Read the model definition and answer for the solid it produces. Units are mm, in the model's axes. A direction names the side the tool comes from. Give positions to 0.01 mm unless a question says otherwise; leave off trailing zeros. Order: outer loops, then holes, each group sorted by start corner. A loop starts at its lowest first (then second) coordinate and runs counter-clockwise, first axis right, second up. Notation, with made-up numbers: (65, -17) - (93, -17) arc R23 ccw to (93, 5) - close; hole circle Ø8 at (-26, -25.5). An arc over 180 degrees is marked (long way). Write each question's results on one line, items separated by ' | '. Start each with the question number.
Q1. Flat-ended cylindrical pins translate along their axes: P1, Ø2, axis at x = -0.5, y = 6, coming from the -Z side; P2, Ø3, axis at x = -19, z = 16.5, coming from the +Y side; P3, Ø5.5, axis at x = 0.5, z = 14, coming from the +Y side. Find the tip coordinate at first contact, or state that the pin passes through.
Q2. For a pull along Y with two mould halves and no side action, classify faces 1 (the face through (0, -7.5, 14)), 2 (the face through (-20, -3, 9)), 3 (the face through (0, 6, 17)), 4 (the face through (20, -2, 9)) as +Y half, -Y half, draft (parallel to the pull), parting line (faces both ways), or undercut.
Q3. A tool of negligible diameter and unlimited length cuts with its end or side. For faces 5 (the face through (20, -2.5, 18)), 6 (the face through (-12.215, -0.105, 11.699)), 7 (the face through (5, 6, 14)), 8 (the face through (24.9, 2.6, 23)), from which of +Z, -Z, +X, -X, +Y, -Y can it reach the whole face along a straight path? Write none if from no direction.
Q4. Find section D-D on z = 12.5. Give the vertices of the cut face in (x, y).
Q5. Find the intervals of material crossed by line 1 along X through (y, z) = (3.25, 18); line 2 along Z through (x, y) = (20, 2.75); line 3 along Y through (x, z) = (-20, 7), in increasing order. Write a range as from..to.
Q6. Find section C-C on x = -7. Give the vertices of the cut face in (y, z).
Q7. Find section B-B on y = 0.75. Give the vertices of the cut face in (x, z).
Q8. Find section A-A on z = 7.75. Give the vertices of the cut face in (x, y), and give its area (3 significant figures).
from build123d import *

# Parameters (mm, degrees)
SKETCH_1_W                = 54
SKETCH_1_H                = 15
EXTRUDE_1_DEPTH           = 25
SKETCH_2_R                = 3
CUT_EXTRUDE_4_DEPTH       = 10
SKETCH_3_R                = 2
CUT_EXTRUDE_5_DEPTH       = 9
FILLET_1_R                = 7
FILLET_2_R                = 5
CHAMFER_1_SIZE            = 0.5
CUT_EXTRUDE_11_DEPTH      = 40.736632973
CUT_EXTRUDE_11_DEPTH_BACK = 40.736632973
CUT_EXTRUDE_12_DEPTH      = 4


with BuildPart() as part:
    # 草图1 → 凸台-拉伸1 (new body)
    with BuildSketch(Plane.XY):
        Rectangle(SKETCH_1_W, SKETCH_1_H)
    extrude(amount=EXTRUDE_1_DEPTH)

    # 草图2 → 切除-拉伸4 (cut)
    with BuildSketch(Plane.XZ.offset(-7.5)):
        with Locations(Location((-20, 18, 0), (0, 0, 270))):
            Circle(SKETCH_2_R)
        with Locations(Location((20, 18, 0), (0, 0, 90))):
            Circle(SKETCH_2_R)
    extrude(amount=CUT_EXTRUDE_4_DEPTH, mode=Mode.SUBTRACT)

    # 草图3 → 切除-拉伸5 (cut)
    with BuildSketch(Plane(origin=(0, 0, 0), x_dir=(-1, 0, 0), z_dir=(0, 0, -1))):
        with Locations((-20, -2.5)):
            Circle(SKETCH_3_R)
        with Locations(Location((20, -2.5, 0), (0, 0, 180))):
            Circle(SKETCH_3_R)
    extrude(amount=-CUT_EXTRUDE_5_DEPTH, mode=Mode.SUBTRACT)

    # 圆角1
    fillet_1_edges = [part.edges().sort_by_distance(p)[0] for p in [
        (-27, 0, 25),
        (27, 0, 25),
    ]]
    fillet(fillet_1_edges, radius=FILLET_1_R)

    # 圆角2
    fillet_2_edges = [part.edges().sort_by_distance(p)[0] for p in [
        (0, -7.5, 25),
        (27, -7.5, 9),
        (-27, -7.5, 9),
        (-24.949747468, -7.5, 22.949747468),
        (24.949747468, -7.5, 22.949747468),
    ]]
    fillet(fillet_2_edges, radius=FILLET_2_R)

    # 倒角1
    chamfer_1_edges = [part.edges().sort_by_distance(p)[0] for p in [
        (-20, 7.5, 21),
        (20, 7.5, 15),
    ]]
    chamfer(chamfer_1_edges, length=CHAMFER_1_SIZE)

    # 草图4 → 切除-拉伸11 (cut, two sides: drawn at the far end of the back side and taken through both)
    with BuildSketch(Plane(origin=(0, 7.5, 0), x_dir=(1, 0, 0), z_dir=(0, 1, 0)).offset(-CUT_EXTRUDE_11_DEPTH_BACK)):
        with BuildLine():
            Line((-11.5, -12), (11.5, -12))
            ThreePointArc((11.5, -12), (12.207106781, -11.707106781), (12.5, -11))
            Line((12.5, -11), (12.5, 3))
            ThreePointArc((12.5, 3), (12.207106781, 3.707106781), (11.5, 4))
            Line((11.5, 4), (-11.5, 4))
            ThreePointArc((-11.5, 4), (-12.207106781, 3.707106781), (-12.5, 3))
            Line((-12.5, 3), (-12.5, -11))
            ThreePointArc((-12.5, -11), (-12.207106781, -11.707106781), (-11.5, -12))
        make_face()
    extrude(amount=CUT_EXTRUDE_11_DEPTH + CUT_EXTRUDE_11_DEPTH_BACK, mode=Mode.SUBTRACT)

    # 草图5 → 切除-拉伸12 (cut)
    with BuildSketch(Plane(origin=(0, 7.5, 0), x_dir=(1, 0, 0), z_dir=(0, 1, 0))):
        with BuildLine():
            Line((-4, -17), (4, -17))
            ThreePointArc((4, -17), (4.707106781, -16.707106781), (5, -16))
            Line((5, -16), (5, -12))
            Line((5, -12), (-5, -12))
            Line((-5, -12), (-5, -16))
            ThreePointArc((-5, -16), (-4.707106781, -16.707106781), (-4, -17))
        make_face()
    extrude(amount=-CUT_EXTRUDE_12_DEPTH, mode=Mode.SUBTRACT)


solid = part.part
Working result:
1) P1: z = 17 | P2: y = 7.3 | P3: y = 3.5
2) face 1: -Y half | face 2: undercut | face 3: draft | face 4: undercut
3) face 5: +Y | face 6: -Z, +Y, -Y | face 7: -Z, +Y | face 8: +Z, +X, +Y, -Y
4) outline: (-27, -2.5) arc R5 ccw to (-22, -7.5) - (22, -7.5) arc R5 ccw to (27, -2.5) - (27, 7.5) - (5, 7.5) - (5, 3.5) - (-5, 3.5) - (-5, 7.5) - (-27, 7.5) - close
5) line 1: -27..-23, -17..17, 23..27 | line 2: 0..15, 21..25 | line 3: -7.5..-4.5, -0.5..7.5
6) outline: (-7.5, 12) - (7.5, 12) - (7.5, 25) - (-2.5, 25) arc R5 ccw to (-7.5, 20) - close
7) outline: (-27, 0) - (-12.5, 0) - (-12.5, 11) arc R1 cw to (-11.5, 12) - (11.5, 12) arc R1 cw to (12.5, 11) - (12.5, 0) - (27, 0) - (27, 18) arc R7 ccw to (20, 25) - (-20, 25) arc R7 ccw to (-27, 18) - close; hole circle Ø6 at (-20, 18); hole circle Ø6 at (20, 18)
8) outline: (-27, -2.5) arc R5 ccw to (-22, -7.5) - (-12.5, -7.5) - (-12.5, 7.5) - (-27, 7.5) - close; (12.5, -7.5) - (22, -7.5) arc R5 ccw to (27, -2.5) - (27, 7.5) - (12.5, 7.5) - close; hole circle Ø4 at (-20, -2.5); hole circle Ø4 at (20, -2.5) | area: 399 mm²
